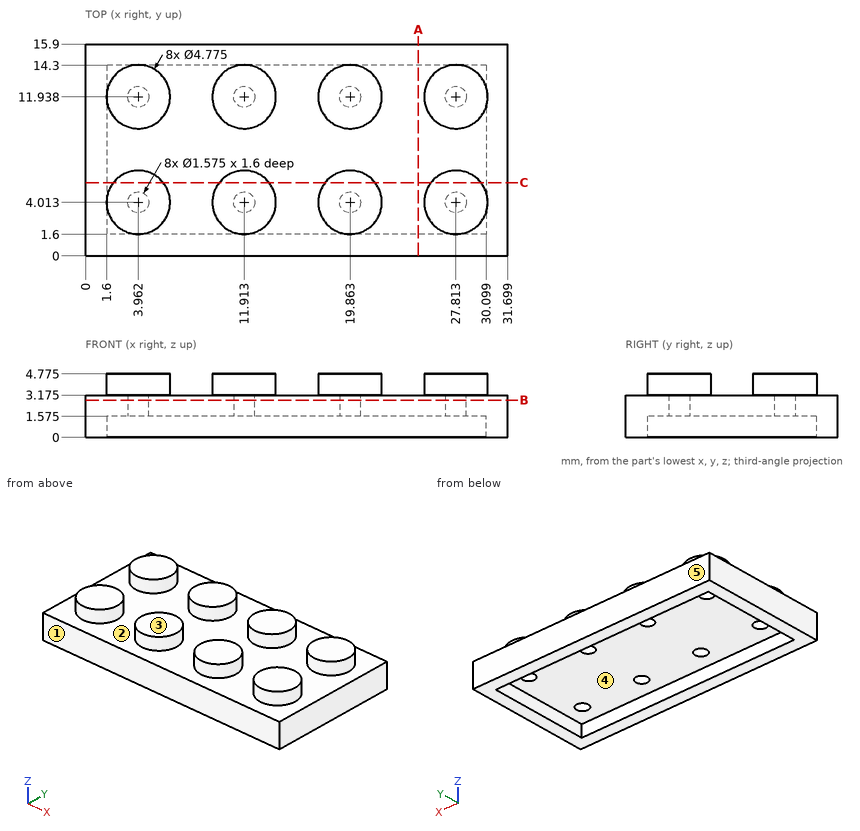
Drawing for the job (mm, zero at the part's lowest x, y, z). A direction names the side the tool comes from. Round coordinates to 2 decimals unless told otherwise and drop trailing zeros. Write each loop counter-clockwise with the first axis right and the second up, starting at its lowest first coordinate (ties: lowest second). Pieces come first, ordered by that corner, then holes.
Item 1: Drop flat-ended pins along their axis: pin 1 Ø0.5 at (x, y) = (20, 4) entering from -Z (3 decimals); pin 2 Ø1.7 at (x, y) = (4, 4.5) entering from -Z (1 decimal); pin 3 Ø3 at (x, y) = (23.5, 2) entering from +Z (3 decimals). Give the stop position or say it passes through.
Filled in:
pin 1: stops at z = 3.175
pin 2: stops at z = 1.6
pin 3: stops at z = 3.175
Item 2: Tool access for the marked faces 1 and 2: list every direction of +Z, -Z, +X, -X, +Y, -Y with a clear straight run to the whole face (end or side of a thin tool).
Filled in:
face 1: +Z, -Z, +X, -X, -Y
face 2: +Z
Item 3: Band-saw the part on C-C on y = 5.5. Write the cut outline in (x, z) (1 decimal).
Filled in:
outline: (0, 0) - (1.6, 0) - (1.6, 1.6) - (30.1, 1.6) - (30.1, 0) - (31.7, 0) - (31.7, 3.2) - (29.7, 3.2) - (29.7, 4.8) - (25.9, 4.8) - (25.9, 3.2) - (21.7, 3.2) - (21.7, 4.8) - (18, 4.8) - (18, 3.2) - (13.8, 3.2) - (13.8, 4.8) - (10, 4.8) - (10, 3.2) - (5.8, 3.2) - (5.8, 4.8) - (2.1, 4.8) - (2.1, 3.2) - (0, 3.2) - close
Item 4: Mould opens along Y. For the marked faces 3, 4 and 5 say: released by +Y, released by -Y, zero draft, split by the parting line, or undercut.
Filled in:
face 3: zero draft
face 4: undercut
face 5: released by +Y
Item 5: Drill centre lines: L1, parallel to X at y = 12, z = 1.7; L2, parallel to X at y = 11.5, z = 0.85; L3, parallel to Y at x = 10, z = 0.4. Where is each one in solid material? Low to high.
Filled in:
L1: x = 0 to 3.18, 4.75 to 11.13, 12.7 to 19.08, 20.65 to 27.03, 28.6 to 31.7
L2: x = 0 to 1.6, 30.1 to 31.7
L3: y = 0 to 1.6, 14.3 to 15.9
Item 6: Band-saw the part on B-B on z = 2.8. Give the number of separate pieces and of enclosed holes in the cut face.
Filled in:
separate pieces: 1
enclosed holes: 8
Item 7: Band-saw the part on A-A on x = 25. Write the cut outline in (y, z) (1 decimal).
Filled in:
outline: (0, 0) - (1.6, 0) - (1.6, 1.6) - (14.3, 1.6) - (14.3, 0) - (15.9, 0) - (15.9, 3.2) - (0, 3.2) - close
